```python
from build123d import *

# Parameters (mm, degrees)
F0_W     = 50
F0_H     = 70
F1_DEPTH = 20
F3_D     = 10
F3_DEPTH = 100
F5_DEPTH = 20


with BuildPart() as f1:
    # F0 (on Right) → F1 (new body)
    with BuildSketch(Plane.YZ):
        with Locations((25, 35)):
            Rectangle(F0_W, F0_H)
    extrude(amount=F1_DEPTH)

    # F3
    with Locations(Plane.YZ.offset(20)):
        with Locations((25, 20), (25, 50)):
            Hole(F3_D / 2, depth=F3_DEPTH)

    # F4 (on face) → F5 (join)
    with BuildSketch(Plane.YZ.offset(20)):
        Polygon((-22.037402, -11.649207), (0, 0), (0, 70), (50, 70), (50, 0), (185.781255, 10.607836), (197.686195, 42.699385), (-30.06028, 102.22403), (-87.773323, 34.417696), (-37.824381, -39.59991), align=None)
    extrude(amount=-F5_DEPTH)


solid = f1.part
```
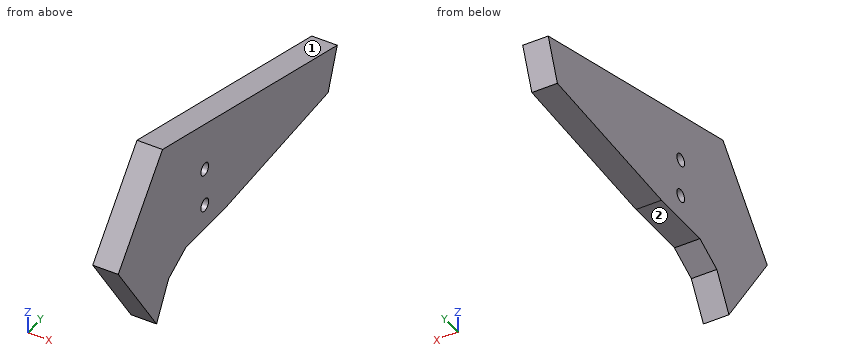
Geometry check sheet. Reference: the model listing, model coordinates, mm. Face numbers are marked on the shaded views. A direction names the side the tool comes from. Coordinates: 2 decimals unless noted, no trailing zeros. Write each loop counter-clockwise with the first axis right and the second up, starting at its lowest first coordinate (ties: lowest second). Pieces come first, ordered by that corner, then holes. Notation, with made-up numbers: M 17,6 L 63,6 A23 cw 63,32 Z; hole C 24.25,66.5 d2. An arc over 180 degrees is marked long. Use one line per item in the form item = value. Start each with the question number.
1) Section check D-D on z = 20. Enter the section's corners in (x, y), and give its area (3 significant figures).
2) Thickness scan on probe 1 along Z at (x, y) = (9.5, 25); probe 2 along Z at (x, y) = (11.5, 21.5); probe 3 along Y at (x, z) = (5.5, 25.5). Record the ranges inside material, lowest first. Write a range as from..to.
3) Section check C-C on x = 9.25. Enter the section's corners in (y, z).
4) Go/stop test with flat-tipped pins: pin 1 Ø1.5 at (x, y) = (6.5, 57) entering from +Z; pin 2 Ø8 at (y, z) = (25, 50) entering from -X; pin 3 Ø6 at (x, y) = (6, 29) entering from -Z; pin 4 Ø3 at (x, y) = (15, -24) entering from +Z. Record where each tip stops, or that it passes through.
5) Set-up check for the marked faces 1 and 2: record each of +Z, -Z, +X, -X, +Y, -Y from which the full face is reachable in a straight line by a thin tool's end or side.
6) Section check B-B on z = 50. Enter the section's corners in (x, y).
7) Section check A-A on y = 25. Enter the section's corners in (x, z), and give its area (3 significant figures).
Responses:
q1.outline = M 0,-78.04 L 20,-78.04 L 20,20 L 0,20 Z; M 0,30 L 20,30 L 20,189.27 L 0,189.27 Z
q1.area = 5,150 mm2
q2.probe_1 = 0..15, 25..45, 55..87.83
q2.probe_2 = 0..16.43, 23.57..46.43, 53.57..88.75
q2.probe_3 = -81.76..191.31
q3.outline = M -87.77,34.42 L -37.82,-39.6 L -22.04,-11.65 L 0,0 L 50,0 L 185.78,10.61 L 197.69,42.7 L -30.06,102.22 Z; hole C 25,20 d10; hole C 25,50 d10
q4.pin_1 = 79.67
q4.pin_2 = through
q4.pin_3 = 0
q4.pin_4 = 101.03
q5.face_1 = +Z, +X, -X, +Y
q5.face_2 = -Z, +X, -X, +Y
q6.outline = M 0,-74.51 L 20,-74.51 L 20,20 L 0,20 Z; M 0,30 L 20,30 L 20,169.75 L 0,169.75 Z
q7.outline = M 0,0 L 20,0 L 20,15 L 0,15 Z; M 0,25 L 20,25 L 20,45 L 0,45 Z; M 0,55 L 20,55 L 20,87.83 L 0,87.83 Z
q7.area = 1,360 mm2
